Autodesk Inventor part; units mm, degrees
ref_plane "YZ Plane" through (0, 0, 0) normal (1, 0, 0) x (0, 1, 0)
ref_plane "XZ Plane" through (0, 0, 0) normal (0, 1, 0) x (-1, 0, 0)
ref_plane "XY Plane" through (0, 0, 0) normal (0, 0, 1) x (1, 0, 0)
sketch "スケッチ1" plane through (0, 0, 0) normal (0, 0, 1) x (1, 0, 0)
  line L0 (0, 0) -> (20, 0)
  line L1 (20, 0) -> (20, 30)
  line L2 (20, 30) -> (0, 30)
  line L3 (0, 30) -> (0, 0)
  dimension "d0" = 20
  dimension "d1" = 30
extrude "押し出し1" add sketch "スケッチ1" along normal blind 600
sketch "スケッチ2" plane through (20, 0, 0) normal (1, 0, 0) x (0, 0, -1)
  circle A0 centre (-510, 15) radius 6.05
  line L0 (0, 30) -> (-600, 30)
  line L1 (-600, 0) -> (-600, 30)
  point P0 (0, 0)
  dimension "d4" = 12.1
  dimension "d5" = 15
  dimension "d6" = 90
extrude "押し出し2" cut sketch "スケッチ2" against normal blind 600
sketch "スケッチ3" plane through (20, 0, 0) normal (1, 0, 0) x (0, 0, -1)
  line L0 (0, 30) -> (-600, 30)
  line L1 (0, 0) -> (0, 30)
  point P0 (-10, 22)
  point P1 (-10, 14)
  dimension "d9" = 8
  dimension "d10" = 10
  dimension "d11" = 8
  dimension "d12" = 10
hole "穴1" at (20, 22, 10) at (20, 14, 10) direction (-1, 0, 0) diameter 3.2 end through all
sketch "スケッチ5" plane through (20, 0, 0) normal (1, 0, 0) x (0, 0, -1)
  circle A0 centre (-510, 15) radius 6.05
  circle A1 centre (-510, 15) radius 10 construction
  point P0 (0, 0)
  point P1 (-520, 15)
  point P2 (-500, 15)
  point P3 (-510, 25)
  dimension "d30" = 20
hole "穴3" at (20, 15, 520) at (20, 15, 500) at (20, 25, 510) direction (-1, 0, 0) diameter 3.2 end through all
properties part number "射出_腕_真2"
Work out the finished part from the listing and answer in its coordinate system (mm). Round coordinates to 2 decimals unless told otherwise and drop trailing zeros.
1) Given pin 1 Ø6 at (x, y) = (5.5, 8.5) entering from -Z, flat-ended and moving along its own axis, determine where the tip first touches the part or whether it passes through.
2) Straight lines are drawn through the part: line 1 (Y direction, x = 12.5, z = 10); line 2 (Y direction, x = 16.25, z = 510); line 3 (Y direction, x = 16, z = 500). For each, find the intervals that lie inside material, in ascending order.
3) The mould has two halves that part along Y. Classify faces 1 (the cylindrical face through (10.14, 15.266, 516.044)), 2 (the flat face through (10, 30, 296)), 3 (the flat face through (0, 15, 296)): pulls with the +Y half, pulls with the -Y half, needs draft (parallel to the pull), parting line crosses it, or undercut.
Completed:
1. pin 1: stops at z = 0
2. line 1: y = 0 to 12.4, 15.6 to 20.4, 23.6 to 30
2. line 2: y = 0 to 8.95, 21.05 to 23.4, 26.6 to 30
2. line 3: y = 0 to 13.4, 16.6 to 30
3. face 1: undercut
3. face 2: pulls with the +Y half
3. face 3: needs draft
